```python
from build123d import *

# Parameters (mm, degrees)
SKETCH_10_R         = 12.5
EXTRUDE_5_DEPTH     = 40
CUT_EXTRUDE_1_DEPTH = 11
SKETCH_12_R         = 4.75
CUT_EXTRUDE_2_DEPTH = 18
SKETCH_13_R         = 2.1
CUT_EXTRUDE_3_DEPTH = 20
SKETCH_14_W         = 76
SKETCH_14_H         = 26
EXTRUDE_8_DEPTH     = 8
SKETCH_15_R         = 4.75
CUT_EXTRUDE_4_DEPTH = 8
SKETCH_16_R         = 1.6
CUT_EXTRUDE_5_DEPTH = 26
SKETCH_17_W         = 13
SKETCH_17_H         = 12.15
CUT_EXTRUDE_6_DEPTH = 8
SKETCH_18_R         = 2.05
SKETCH_18_R_2       = 1.6
EXTRUDE_9_DEPTH     = 3.75
EXTRUDE_START       = 3.75
SKETCH_19_R         = 2.05
SKETCH_19_R_2       = 1.6
EXTRUDE_10_DEPTH    = 3.75
SKETCH_20_R         = 2.05
SKETCH_20_R_2       = 1.6
EXTRUDE_11_DEPTH    = 3.75
SKETCH_21_R         = 2.05
SKETCH_21_R_2       = 1.6
EXTRUDE_12_DEPTH    = 3.75
CUT_EXTRUDE_7_DEPTH = 2.5


with BuildPart() as part:
    # 草图10 → 凸台-拉伸5 (new body)
    with BuildSketch(Plane(origin=(0, 0, 0), x_dir=(1, 0, 0), z_dir=(0, 1, 0))):
        with Locations(Location((0, 0, 0), (0, 0, 270))):
            Circle(SKETCH_10_R)
    extrude(amount=EXTRUDE_5_DEPTH)

    # 草图11 → 切除-拉伸1 (cut)
    with BuildSketch(Plane(origin=(0, 0, 0), x_dir=(-1, 0, 0), z_dir=(0, -1, 0))):
        Polygon((5.739953665, -4.542612896), (6.803995, 2.699639243), (1.064041335, 7.242252139), (-5.739953665, 4.542612896), (-6.803995, -2.699639243), (-1.064041335, -7.242252139), align=None)
    extrude(amount=-CUT_EXTRUDE_1_DEPTH, mode=Mode.SUBTRACT)

    # 草图12 → 切除-拉伸2 (cut)
    with BuildSketch(Plane(origin=(0, 40, 0), x_dir=(1, 0, 0), z_dir=(0, 1, 0))):
        with Locations(Location((0, 0, 0), (0, 0, 270))):
            Circle(SKETCH_12_R)
    extrude(amount=-CUT_EXTRUDE_2_DEPTH, mode=Mode.SUBTRACT)

    # 草图13 → 切除-拉伸3 (cut)
    with BuildSketch(Plane(origin=(0, 22, 0), x_dir=(1, 0, 0), z_dir=(0, 1, 0))):
        with Locations(Location((0, 0, 0), (0, 0, 270))):
            Circle(SKETCH_13_R)
    extrude(amount=-CUT_EXTRUDE_3_DEPTH, mode=Mode.SUBTRACT)

    # 草图14 → 凸台-拉伸8 (add)
    with BuildSketch(Plane(origin=(0, 40, 0), x_dir=(1, 0, 0), z_dir=(0, 1, 0))):
        Rectangle(SKETCH_14_W, SKETCH_14_H)
    extrude(amount=EXTRUDE_8_DEPTH)

    # 草图15 → 切除-拉伸4 (cut)
    with BuildSketch(Plane(origin=(0, 48, 0), x_dir=(1, 0, 0), z_dir=(0, 1, 0))):
        with Locations(Location((0, 0, 0), (0, 0, 270))):
            Circle(SKETCH_15_R)
    extrude(amount=-CUT_EXTRUDE_4_DEPTH, mode=Mode.SUBTRACT)

    # 草图16 → 切除-拉伸5 (cut)
    with BuildSketch(Plane.XY.offset(13)):
        with Locations((-33.45, 44)):
            Circle(SKETCH_16_R)
        with Locations((33.45, 44)):
            Circle(SKETCH_16_R)
    extrude(amount=-CUT_EXTRUDE_5_DEPTH, mode=Mode.SUBTRACT)

    # 草图17 → 切除-拉伸6 (cut)
    with BuildSketch(Plane.XZ.offset(-40)):
        with Locations((31.5, 0)):
            Rectangle(SKETCH_17_W, SKETCH_17_H)
        with Locations((-31.5, 0)):
            Rectangle(SKETCH_17_W, SKETCH_17_H)
    extrude(amount=-CUT_EXTRUDE_6_DEPTH, mode=Mode.SUBTRACT)

    # 草图18 → 凸台-拉伸9 (add)
    with BuildSketch(Plane(origin=(0, 0, 6.075), x_dir=(-1, 0, 0), z_dir=(0, 0, -1))):
        with Locations(Location((33.45, 44, 0), (0, 0, 180))):
            Circle(SKETCH_18_R)
        with Locations(Location((33.45, 44, 0), (0, 0, 180))):
            Circle(SKETCH_18_R_2, mode=Mode.SUBTRACT)
    extrude(amount=EXTRUDE_9_DEPTH)

    # 草图19 → 凸台-拉伸10 (add)
    with BuildSketch(Plane.XY.offset(-6.075).offset(EXTRUDE_START)):
        with Locations((-33.45, 44)):
            Circle(SKETCH_19_R)
        with Locations((-33.45, 44)):
            Circle(SKETCH_19_R_2, mode=Mode.SUBTRACT)
    extrude(amount=-EXTRUDE_10_DEPTH)

    # 草图20 → 凸台-拉伸11 (add)
    with BuildSketch(Plane.XY.offset(-6.075).offset(EXTRUDE_START)):
        with Locations(Location((33.45, 44, 0), (0, 0, 180))):
            Circle(SKETCH_20_R)
        with Locations((33.45, 44)):
            Circle(SKETCH_20_R_2, mode=Mode.SUBTRACT)
    extrude(amount=-EXTRUDE_11_DEPTH)

    # 草图21 → 凸台-拉伸12 (add)
    with BuildSketch(Plane(origin=(0, 0, 6.075), x_dir=(-1, 0, 0), z_dir=(0, 0, -1))):
        with Locations((-33.45, 44)):
            Circle(SKETCH_21_R)
        with Locations(Location((-33.45, 44, 0), (0, 0, 180))):
            Circle(SKETCH_21_R_2, mode=Mode.SUBTRACT)
    extrude(amount=EXTRUDE_12_DEPTH)

    # 草图22 → 切除-拉伸7 (cut)
    with BuildSketch(Plane(origin=(0, 0, -13), x_dir=(-1, 0, 0), z_dir=(0, 0, -1))):
        Polygon((-30.05, 44), (-31.75, 46.944486373), (-35.15, 46.944486373), (-36.85, 44), (-35.15, 41.055513627), (-31.75, 41.055513627), align=None)
        Polygon((36.85, 44), (35.15, 46.944486373), (31.75, 46.944486373), (30.05, 44), (31.75, 41.055513627), (35.15, 41.055513627), align=None)
    extrude(amount=-CUT_EXTRUDE_7_DEPTH, mode=Mode.SUBTRACT)


solid = part.part
```
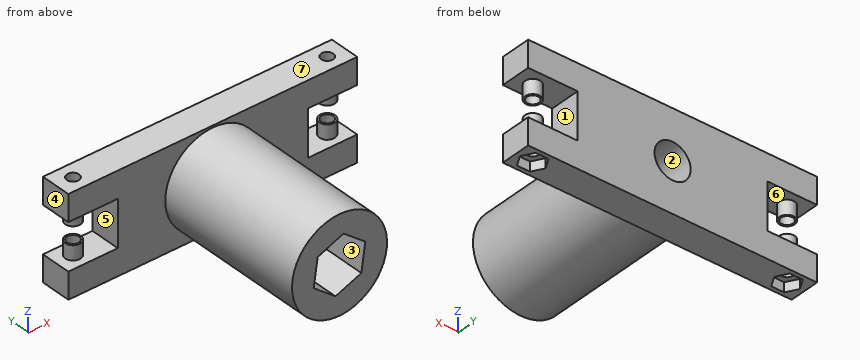
Verification items for the finished model (mm, model axes). Face numbers are marked on the shaded views. A direction names the side the tool comes from. Coordinates: 2 decimals unless noted, no trailing zeros. Loops run counter-clockwise (first coordinate to the right, second up) from the corner with the lowest first, then second, coordinate; pieces in that order, holes last. Notation, with made-up numbers: (-6.5, 16) - (51.5, 16) arc R21 ccw to (51.5, 37) - close; hole circle Ø5 at (-40, 21.25). An arc over 180 degrees is marked (long way). Return JSON: item names as keys, results as strings.
1. Section check C-C, the plane y = 5. Record the boundary of the cut face in (x, z).
Established:
{"outline": "circle Ø25 at (0, 0); hole (-6.8, -2.7) - (-1.06, -7.24) - (5.74, -4.54) - (6.8, 2.7) - (1.06, 7.24) - (-5.74, 4.54) - close"}
2. Section check A-A, the plane z = 3.75. Record the boundary of the cut face in (x, y).
Established:
{"outline": "circle Ø4.1 at (-33.45, 44); (-25, 40) - (-11.92, 40) - (-11.92, 0) - (-5.86, 0) - (-5.86, 11) - (5.48, 11) - (5.48, 0) - (11.92, 0) - (11.92, 40) - (25, 40) - (25, 48) - (2.92, 48) - (2.92, 22) - (-2.92, 22) - (-2.92, 48) - (-25, 48) - close; circle Ø4.1 at (33.45, 44); hole circle Ø3.2 at (-33.45, 44); hole circle Ø3.2 at (33.45, 44)"}
3. Go/stop test with flat-tipped pins: pin 1 (4 mm diameter, centred on x = 33.45, y = 44, fed in from -Z); pin 2 (4 mm diameter, centred on x = 0, y = 36, fed in from +Z); pin 3 (1.5 mm diameter, centred on y = 6, z = 2.5, fed in from +X). Record where each tip stops, or that it passes through.
Established:
{"pin 1": "stops at z = -10.5", "pin 2": "stops at z = 12.5", "pin 3": "stops at x = 12.38"}
4. Section check B-B, the plane x = 33.45. Record the boundary of the cut face in (y, z) (3 decimals), then the cut area to 3 significant figures.
Established:
{"outline": "(40, -13) - (41.056, -13) - (41.056, -10.5) - (42.4, -10.5) - (42.4, -2.325) - (41.95, -2.325) - (41.95, -6.075) - (40, -6.075) - close; (40, 6.075) - (41.95, 6.075) - (41.95, 2.325) - (42.4, 2.325) - (42.4, 13) - (40, 13) - close; (45.6, -10.5) - (46.944, -10.5) - (46.944, -13) - (48, -13) - (48, -6.075) - (46.05, -6.075) - (46.05, -2.325) - (45.6, -2.325) - close; (45.6, 2.325) - (46.05, 2.325) - (46.05, 6.075) - (48, 6.075) - (48, 13) - (45.6, 13) - close", "area": "66.5 mm2"}
5. Tool access check on the marked faces 1, 2 and 3. Record the directions out of +Z, -Z, +X, -X, +Y, -Y that give a thin tool (end or side, any length) a straight path to the whole face; none if there is none.
Established:
{"face 1": "+Y, -Y", "face 2": "+Y", "face 3": "-Y"}
6. Thickness scan on L1, parallel to Y at x = 32, z = -10.75; L2, parallel to Y at x = -33.45, z = -6.75; L3, parallel to Y at x = -16, z = -3. Record the ranges inside material, lowest first.
Established:
{"L1": "y = 40 to 41.06, 46.94 to 48", "L2": "y = 40 to 42.4, 45.6 to 48", "L3": "y = 40 to 48"}
7. Mould release check, pull along X, two halves, no side actions. Record for the marked faces 4, 5, 6 and 7: +X half, -X half, draft (parallel to the pull), parting line (faces both ways), or undercut.
Established:
{"face 4": "-X half", "face 5": "undercut", "face 6": "undercut", "face 7": "draft"}
8. Section check D-D, the plane z = 0. Record the boundary of the cut face in (x, y).
Established:
{"outline": "(-25, 40) - (-12.5, 40) - (-12.5, 0) - (-6.41, 0) - (-6.41, 11) - (-2.1, 11) - (-2.1, 22) - (-4.75, 22) - (-4.75, 48) - (-25, 48) - close; (2.1, 11) - (6.41, 11) - (6.41, 0) - (12.5, 0) - (12.5, 40) - (25, 40) - (25, 48) - (4.75, 48) - (4.75, 22) - (2.1, 22) - close"}
